from build123d import *

# Parameters (mm, degrees)
SKETCH_W        = 192.8
SKETCH_H        = 166
PAD_DEPTH       = 40
SKETCH001_W     = 183.8
SKETCH001_H     = 160
POCKET_DEPTH    = 37
SKETCH002_R     = 1.6
POCKET001_DEPTH = 192.801
POCKET002_DEPTH = 2.6
SKETCH004_R     = 5
POCKET003_DEPTH = 1
SKETCH005_R     = 5
POCKET004_DEPTH = 1
POCKET005_DEPTH = 1.6
FILLET_R        = 3
CHAMFER_SIZE    = 1.5


with BuildPart() as part:
    # Sketch → Pad (new body)
    with BuildSketch(Plane.XY):
        Rectangle(SKETCH_W, SKETCH_H)
    extrude(amount=PAD_DEPTH)

    # Sketch001 (on Face6 of Pad) → Pocket (cut)
    with BuildSketch(Plane.XY.offset(40)):
        Rectangle(SKETCH001_W, SKETCH001_H)
    extrude(amount=-POCKET_DEPTH, mode=Mode.SUBTRACT)

    # Sketch002 (on Face3 of Pocket) → Pocket001 (cut, through all)
    with BuildSketch(Plane.YZ.offset(96.4)):
        with Locations((-71, 9.5)):
            Circle(SKETCH002_R)
        with Locations((-50, 9.5)):
            Circle(SKETCH002_R)
        with Locations((50, 9.5)):
            Circle(SKETCH002_R)
        with Locations((71, 9.5)):
            Circle(SKETCH002_R)
    extrude(amount=-POCKET001_DEPTH, mode=Mode.SUBTRACT)

    # Sketch003 (on Face2 of Pocket001) → Pocket002 (cut)
    with BuildSketch(Plane(origin=(-96.4, 0, 0), x_dir=(0, -1, 0), z_dir=(-1, 0, 0))):
        with BuildLine():
            ThreePointArc((-66.2, 9.5), (-71, 14.3), (-75.8, 9.5))
            Line((-75.8, 9.5), (-75.8, -4.8))
            ThreePointArc((-75.8, -4.8), (-71, -9.6), (-66.2, -4.8))
            Line((-66.2, -4.8), (-66.2, 9.5))
        make_face()
        with BuildLine():
            ThreePointArc((75.8, 9.5), (71, 14.3), (66.2, 9.5))
            Line((66.2, 9.5), (66.2, -4.8))
            ThreePointArc((66.2, -4.8), (71, -9.6), (75.8, -4.8))
            Line((75.8, -4.8), (75.8, 9.5))
        make_face()
    extrude(amount=-POCKET002_DEPTH, mode=Mode.SUBTRACT)

    # Sketch004 (on Face21 of Pocket002) → Pocket003 (cut)
    with BuildSketch(Plane.YZ.offset(-91.9)):
        with Locations((-71, 9.5)):
            Circle(SKETCH004_R)
        with Locations((71, 9.5)):
            Circle(SKETCH004_R)
    extrude(amount=-POCKET003_DEPTH, mode=Mode.SUBTRACT)

    # Sketch005 (on Face23 of Pocket003) → Pocket004 (cut)
    with BuildSketch(Plane(origin=(91.9, 0, 0), x_dir=(0, -1, 0), z_dir=(-1, 0, 0))):
        with Locations((-71, 9.5)):
            Circle(SKETCH005_R)
        with Locations((71, 9.5)):
            Circle(SKETCH005_R)
    extrude(amount=-POCKET004_DEPTH, mode=Mode.SUBTRACT)

    # Sketch006 (on Face3 of Pocket004) → Pocket005 (cut)
    with BuildSketch(Plane.YZ.offset(96.4)):
        with BuildLine():
            ThreePointArc((-66.2, 9.5), (-71, 14.3), (-75.8, 9.5))
            Line((-75.8, 9.5), (-75.8, -4.8))
            ThreePointArc((-75.8, -4.8), (-71, -9.6), (-66.2, -4.8))
            Line((-66.2, -4.8), (-66.2, 9.5))
        make_face()
        with BuildLine():
            ThreePointArc((75.8, 9.5), (71, 14.3), (66.2, 9.5))
            Line((66.2, 9.5), (66.2, -4.8))
            ThreePointArc((66.2, -4.8), (71, -9.6), (75.8, -4.8))
            Line((75.8, -4.8), (75.8, 9.5))
        make_face()
    extrude(amount=-POCKET005_DEPTH, mode=Mode.SUBTRACT)

    # Fillet
    fillet_edges = [part.edges().sort_by_distance(p)[0] for p in [
        (91.9, 80, 21.5),
        (-91.9, 80, 21.5),
        (-91.9, -80, 21.5),
        (91.9, -80, 21.5),
        (91.9, 0, 3),
        (0, -80, 3),
        (-91.9, 0, 3),
        (0, 80, 3),
        (-96.4, 83, 20),
        (-96.4, -83, 20),
        (96.4, -83, 20),
        (96.4, 83, 20),
    ]]
    fillet(fillet_edges, radius=FILLET_R)

    # Chamfer
    chamfer_edges = [part.edges().sort_by_distance(p)[0] for p in [
        (-93.8, -71, 0),
        (-95.1, -66.2, 0),
        (-95.1, -75.8, 0),
        (-95.1, 75.8, 0),
        (-93.8, 71, 0),
        (-95.1, 66.2, 0),
        (94.8, -71, 0),
        (95.6, -66.2, 0),
        (95.6, -75.8, 0),
        (94.8, 71, 0),
        (95.6, 66.2, 0),
        (95.6, 75.8, 0),
    ]]
    chamfer(chamfer_edges, length=CHAMFER_SIZE)


solid = part.part
Model file for the job. Use its own axes, mm. A direction names the side the tool comes from. Give positions to 0.01 mm unless a question says otherwise; leave off trailing zeros. Loops run counter-clockwise (first coordinate to the right, second up) from the corner with the lowest first, then second, coordinate; pieces in that order, holes last.
Item 1: Slice it at A-A (z = 37). Write the cut outline in (x, y), plus the area to 3 significant figures.
Check values:
outline: (-96.4, -80) arc R3 ccw to (-93.4, -83) - (93.4, -83) arc R3 ccw to (96.4, -80) - (96.4, 80) arc R3 ccw to (93.4, 83) - (-93.4, 83) arc R3 ccw to (-96.4, 80) - close; hole (-91.9, -77) arc R3 ccw to (-88.9, -80) - (88.9, -80) arc R3 ccw to (91.9, -77) - (91.9, 77) arc R3 ccw to (88.9, 80) - (-88.9, 80) arc R3 ccw to (-91.9, 77) - close
area: 2,600 mm2
Item 2: Which spindle directions (+Z, -Z, +X, -X, +Y, -Y) get a long thin tool onto all of the face, cutting with end or side? Do faces 5 (the face through (95.6, -70.9, 14.3)), 6 (the face through (-0.4, 80.3, 40)), 7 (the face through (-95.1, 70.9, 14.3)), 8 (the face through (-92.9, 70, 11)), 9 (the face through (91.9, -1, 23)). Say none if no direction does.
Check values:
face 5: -Z, +X
face 6: +Z, +X, -X, +Y, -Y
face 7: -Z, -X
face 8: none
face 9: +Z
Item 3: Slice it at B-B (x = 74). Write the cut outline in (y, z).
Check values:
outline: (-83, 0) - (83, 0) - (83, 40) - (80, 40) - (80, 6) arc R3 cw to (77, 3) - (-77, 3) arc R3 cw to (-80, 6) - (-80, 40) - (-83, 40) - close
Item 4: Drill centre lines: line 1 along Y through (x, z) = (93, 9); line 2 along X through (y, z) = (-2, 16); line 3 along Y through (x, z) = (-19, 32). Where is each one in solid material? Low to high.
Check values:
line 1: y = -83 to -72.52, -69.48 to -51.52, -48.48 to 48.48, 51.52 to 69.48, 72.52 to 83
line 2: x = -96.4 to -91.9, 91.9 to 96.4
line 3: y = -83 to -80, 80 to 83
Item 5: Slice it at C-C (y = 59). Write the cut outline in (x, z).
Check values:
outline: (-96.4, 0) - (96.4, 0) - (96.4, 40) - (91.9, 40) - (91.9, 6) arc R3 cw to (88.9, 3) - (-88.9, 3) arc R3 cw to (-91.9, 6) - (-91.9, 40) - (-96.4, 40) - close
Item 6: Mould opens along Y. For faces 1 (the face through (-95.1, -71.1, 14.3)), 2 (the face through (-1, 1, 0)), 3 (the face through (-1, -83, 20)), 4 (the face through (-1, 1, 3)) say: +Y half, -Y half, draft (parallel to the pull), parting line (faces both ways), or undercut.
Check values:
face 1: undercut
face 2: draft
face 3: -Y half
face 4: undercut
Item 7: Drop flat-ended pins along their axis: P1, Ø5, axis at y = -70.5, z = 10, coming from the +X side; P2, Ø2, axis at x = -95, z = 4.5, coming from the +Y side; P3, Ø0.5, axis at x = 95.5, z = 7, coming from the +Y side; P4, Ø16, axis at y = 71, z = 9.5, coming from the -X side. Give the stop position or say it passes through.
Check values:
P1: stops at x = 94.8
P2: stops at y = 82.94
P3: stops at y = 82.36
P4: stops at x = -96.4
